Source: three-view drawing plus pictorial views. Frame: mm from the lowest corner of the part. A direction names the side the tool comes from. Give positions to 0.01 mm unless a question says otherwise; leave off trailing zeros. Loops run counter-clockwise (first coordinate to the right, second up) from the corner with the lowest first, then second, coordinate; pieces in that order, holes last. Notation, with made-up numbers: (-3.5, -7) -> (39.5, -7) arc R10 ccw to (39.5, 8) -> close; hole circle Ø11 at (-3, 30). An arc over 180 degrees is marked (long way). Put each result on its own line as item: value.
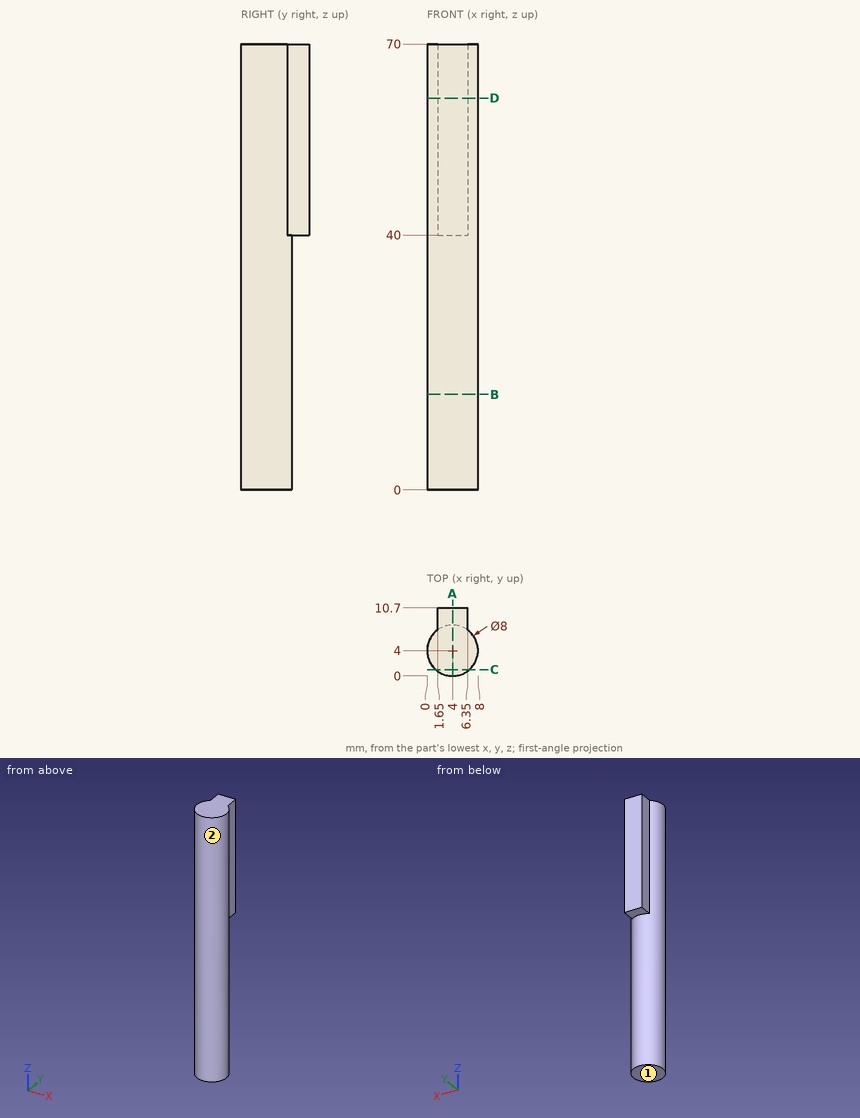
(1) Section A-A on x = 4. Return loops of the section in (y, z).
Calculated:
outline: (0, 0) -> (8, 0) -> (8, 40) -> (10.7, 40) -> (10.7, 70) -> (0, 70) -> close
(2) Section D-D on z = 61.5. Return loops of the section in (x, y), then the cut area to 3 significant figures.
Calculated:
outline: (1.65, 7.24) arc R4 ccw (long way) to (6.35, 7.24) -> (6.35, 10.7) -> (1.65, 10.7) -> close
area: 64.1 mm²
(3) Reachability of the marked faces 1 and 2 from +Z, -Z, +X, -X, +Y, -Y: full face, straight path, thin tool, end or side. Return the list, or none.
Calculated:
face 1: -Z, +X, -X, +Y, -Y
face 2: -Z
(4) Section C-C on y = 1. Return loops of the section in (x, z).
Calculated:
outline: (1.35, 0) -> (6.65, 0) -> (6.65, 70) -> (1.35, 70) -> close
(5) Section B-B on z = 15. Return loops of the section in (x, y), then the cut area to 3 significant figures.
Calculated:
outline: circle Ø8 at (4, 4)
area: 50.3 mm²
(6) First-contact query: P1, Ø4, axis at y = 8, z = 50, coming from the +X side; P2, Ø1.5, axis at x = 5, z = 21, coming from the -Y side; P3, Ø2, axis at y = 8, z = 25.5, coming from the +X side. Flat tips, straight axial feed; report the tip coordinate or a pass-through.
Calculated:
P1: stops at x = 7.46
P2: stops at y = 0.01
P3: stops at x = 6.65
(7) Line query: probe 1 along X at (y, z) = (8.5, 53); probe 2 along Y at (x, z) = (6, 33.5). Output: solid intervals per line, ascending. Write a range as from..to.
Calculated:
probe 1: x = 1.65..6.35
probe 2: y = 0.54..7.46
